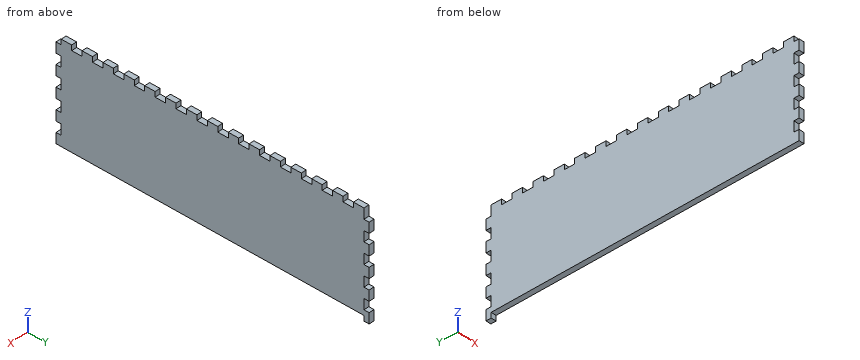
```python
from build123d import *

# Parameters (mm, degrees)
SKETCH012_W             = 90
SKETCH012_H             = 290
PAD010_DEPTH            = 5
SKETCH042_W             = 10
SKETCH042_H             = 5
PAD031_DEPTH            = 5
LINEARPATTERN022_COUNT  = 15
LINEARPATTERN022_PITCH  = 20
SKETCH043_W             = 10
SKETCH043_H             = 5
PAD032_DEPTH            = 5
LINEARPATTERN023_COUNT  = 5
LINEARPATTERN023_PITCH  = 20
SKETCH044_W             = 10
SKETCH044_H             = 5
PAD033_DEPTH            = 5
LINEARPATTERN024_COUNT  = 5
LINEARPATTERN024_PITCH  = 20
BODY010_PLACEMENT_ANGLE = 90


with BuildPart() as part:
    # Sketch012 → Pad010 (new body)
    with BuildSketch(Plane.XY):
        Rectangle(SKETCH012_W, SKETCH012_H)
    extrude(amount=PAD010_DEPTH)

    # Sketch042 (on DatumPlane) → Pad031 (join)
    with BuildSketch(Plane.YZ.offset(45)):
        with Locations((-140, 2.5)):
            Rectangle(SKETCH042_W, SKETCH042_H)
    pad031 = extrude(amount=PAD031_DEPTH)

    # LinearPattern022: Pad031 ×15
    with Locations(*[(0, i * LINEARPATTERN022_PITCH, 0) for i in range(1, LINEARPATTERN022_COUNT)]):
        add(pad031)

    # Sketch043 (on DatumPlane) → Pad032 (join)
    with BuildSketch(Plane(origin=(0, 145, 0), x_dir=(-1, 0, 0), z_dir=(0, 1, 0))):
        with Locations((-35, 2.5)):
            Rectangle(SKETCH043_W, SKETCH043_H)
    pad032 = extrude(amount=PAD032_DEPTH)

    # LinearPattern023: Pad032 ×5
    with Locations(*[(-i * LINEARPATTERN023_PITCH, 0, 0) for i in range(1, LINEARPATTERN023_COUNT)]):
        add(pad032)

    # Sketch044 (on DatumPlane) → Pad033 (join)
    with BuildSketch(Plane.XZ.offset(145)):
        with Locations((-40, 2.5)):
            Rectangle(SKETCH044_W, SKETCH044_H)
    pad033 = extrude(amount=PAD033_DEPTH)

    # LinearPattern024: Pad033 ×5
    with Locations(*[(i * LINEARPATTERN024_PITCH, 0, 0) for i in range(1, LINEARPATTERN024_COUNT)]):
        add(pad033)


with BuildPart() as part_1:
    # Body010 placement: moved
    add(part.part.moved(Location((0, 0, 155))).rotate(Axis((0, 0, 155), (0, -1, 0)), BODY010_PLACEMENT_ANGLE))


solid = part_1.part
```
For this review, take the finished solid that the model builds, in its own axes (mm). Coordinates: 2 decimals unless noted, no trailing zeros. Loops run counter-clockwise (first coordinate to the right, second up) from the corner with the lowest first, then second, coordinate; pieces in that order, holes last.
1. Add section A-A, the plane y = -51. Give the boundary of the cut face in (x, z), then the cut area to 3 significant figures.
2. Insertion check: P1, Ø1.5, axis at x = -3, z = 201.5, coming from the -Y side; P2, Ø1.5, axis at x = -2.5, y = -26.5, coming from the -Z side; P3, Ø1.5, axis at x = -1.5, z = 201.5, coming from the +Y side. Each pin has a flat end and moves straight along its axis. Give the tip position at first contact, or say it passes through.
3. For line 1 (Z direction, x = -3.45, y = -133); line 2 (Y direction, x = -2, z = 116.5); line 3 (Z direction, x = -1.75, y = 122), list the stretches that pass through material, from the lowest coordinate up.
Result:
1. outline: (-5, 110) - (0, 110) - (0, 200) - (-5, 200) - close
1. area: 450 mm2
2. P1: stops at y = -145
2. P2: stops at z = 110
2. P3: stops at y = 145
3. line 1: z = 110 to 200
3. line 2: y = -150 to 145
3. line 3: z = 110 to 205
